Autodesk Inventor part; units mm, degrees
ref_plane "YZ Plane" through (0, 0, 0) normal (1, 0, 0) x (0, 1, 0)
ref_plane "XZ Plane" through (0, 0, 0) normal (0, 1, 0) x (-1, 0, 0)
ref_plane "XY Plane" through (0, 0, 0) normal (0, 0, 1) x (1, 0, 0)
sketch "Sketch4" plane through (0, 0, 0) normal (0, 0, 1) x (1, 0, 0)
  line L0 (1.3586, -0.1628) -> (1.3586, 19.8372)
  line L1 (1.3586, 19.8372) -> (26.3586, 19.8372)
  line L2 (26.3586, 19.8372) -> (36.8586, 14.8372)
  line L3 (36.8586, 14.8372) -> (173.3586, 14.8372)
  line L4 (173.3586, 14.8372) -> (173.3586, -50.1628)
  line L5 (173.3586, -50.1628) -> (153.3586, -50.1628)
  line L6 (153.3586, -50.1628) -> (153.3586, -5.1628)
  line L7 (153.3586, -5.1628) -> (36.8586, -5.1628)
  line L8 (36.8586, -5.1628) -> (26.3586, -0.1628)
  line L9 (26.3586, -0.1628) -> (1.3586, -0.1628)
  dimension "d55" = 20
  dimension "d56" = 25
  dimension "d57" = 5
  dimension "d58" = 20
  dimension "d59" = 45
  dimension "d60" = 152
  dimension "d61" = 10.5
extrude "Arm Base" add sketch "Sketch4" along normal blind 10
sketch "Sketch5" plane through (0, 0, 10) normal (0, 0, 1) x (1, 0, 0)
  line L0 (153.3586, -50.1628) -> (173.3586, -50.1628)
  line L1 (153.3586, -5.1628) -> (153.3586, -50.1628)
  point P0 (163.3586, -40.1628)
  dimension "d62" = 10
  dimension "d63" = 10
hole "Pivot Holes" at (163.3586, -40.1628, 10) direction (0, 0, -1) diameter 8 end through all
sketch "Sketch6" plane through (0, 0, 10) normal (0, 0, 1) x (1, 0, 0)
  line L0 (7.8586, 13.3372) -> (14.8586, 13.3372)
  line L1 (14.8586, 13.3372) -> (14.8586, 6.3372)
  line L2 (14.8586, 6.3372) -> (7.8586, 6.3372)
  line L3 (7.8586, 6.3372) -> (7.8586, 13.3372)
  line L4 (1.3586, 19.8372) -> (1.3586, -0.1628)
  point P0 (0, 0)
  point P1 (7.8586, 9.8372)
  point P2 (1.3586, 9.8372)
  dimension "d48" = 7
  dimension "d64" = 6.5
extrude "Extrusion5" cut sketch "Sketch6" against normal up to next
fillet "Fillet2" radius 10 5 edges at (1.3586, -0.1628, 5) (1.3586, 19.8372, 5) (173.3586, -50.1628, 5) (153.3586, -50.1628, 5) (173.3586, 14.8372, 5)
fillet "Fillet3" radius 2 26 edges at (170.4298, 11.9084, 10) (173.3586, -17.6628, 10) (170.4298, -47.234, 10) (153.3586, -22.6631, 10) (100.1089, 14.8372, 10) (95.1086, -5.1628, 10) (170.4298, -47.234, 0) (153.3586, -22.6631, 0) (170.4298, 11.9084, 0) (100.1089, 14.8372, 0) (173.3586, -17.6628, 0) (95.1086, -5.1628, 0) (18.8584, -0.1628, 0) (18.8584, 19.8372, 0) (4.2874, 2.766, 0) (18.8584, 19.8372, 10) (18.8584, -0.1628, 10) (4.2874, 2.766, 10) (31.6086, 17.3372, 10) (31.6086, -2.6628, 10) (31.6086, -2.6628, 0) (31.6086, 17.3372, 0) (26.3586, 19.8372, 5) (36.8586, 14.8372, 5) (26.3586, -0.1628, 5) (36.8586, -5.1628, 5)
fillet "Fillet4" radius 1 2 edges at (163.3586, -36.1628, 10) (163.3586, -36.1628, 0)
fillet "Fillet5" radius 1 8 edges at (7.8586, 9.8372, 10) (11.3586, 13.3372, 10) (14.8586, 9.8372, 10) (11.3586, 6.3372, 10) (7.8586, 9.8372, 0) (11.3586, 6.3372, 0) (14.8586, 9.8372, 0) (11.3586, 13.3372, 0)
properties part number "Lift Arm Lower"
The listing builds one solid part. Answer for the finished solid, in the listing's coordinates (mm). A direction names the side the tool comes from. Coordinates: 2 decimals unless noted, no trailing zeros. Write each loop counter-clockwise with the first axis right and the second up, starting at its lowest first coordinate (ties: lowest second). Pieces come first, ordered by that corner, then holes. Notation, with made-up numbers: (59, 74) - (79, 74) arc R17 ccw to (79, 78) - close; hole circle Ø8 at (-12.5, 44.5). An arc over 180 degrees is marked (long way). Return JSON: item names as keys, results as strings. Group by question number.
Q1. Find the intervals of material crossed by line 1 along X through (y, z) = (-40, 3.75); line 2 along X through (y, z) = (-6.5, 7.25); line 3 along X through (y, z) = (-36.5, 2.25), in increasing order. Write a range as [from, to].
Q2. Flat-ended cylindrical pins translate along their axes: pin 1 Ø5 at (x, z) = (92.5, 6) entering from -Y; pin 2 Ø1.8 at (y, z) = (-21, 6) entering from -X; pin 3 Ø3.5 at (x, z) = (13, 5.5) entering from -Y; pin 4 Ø5.5 at (y, z) = (9.5, 5) entering from -X. Find the tip coordinate at first contact, or state that the pin passes through.
Q3. The part is cut by section B-B on z = 5.5. State how many separate pieces and enclosed holes the cut face has, and give its area (3 significant figures).
Q4. Which of the six approach directions +Z, -Z, +X, -X, +Y, -Y give full straight-line access (tool end or side, diameter ignored) to faces 5 (the cylindrical face through (31.8, -2.09, 0.57)), 6 (the flat face through (153.359, -23, 5))?
Q5. The part is cut by section A-A on y = -16. Write down the section's boundary in (x, z).
Q6. For a pull along Y with two mould halves and no side action, classify faces 1 (the flat face through (31.676, -2.695, 4.958)), 2 (the cylindrical face through (167.263, -39.296, 4.944)), 3 (the cylindrical face through (31.43, 16.79, 9.4)), 4 (the flat face through (11, 6.337, 5)) as +Y half, -Y half, draft (parallel to the pull), parting line (faces both ways), or undercut.
Q7. The part is cut by section C-C on x = 18.5. Write down the section's boundary in (y, z), and give its area (3 significant figures).
Evaluation:
{
 "1": {"line 1": "x = [153.36, 159.36], [167.36, 173.36]", "line 2": "x = [153.36, 173.36]", "line 3": "x = [153.36, 161.75], [164.97, 173.36]"},
 "2": {"pin 1": "stops at y = -5.16", "pin 2": "stops at x = 153.36", "pin 3": "stops at y = -0.16", "pin 4": "stops at x = 1.36"},
 "3": {"separate pieces": "1", "enclosed holes": "2", "area": "4,130 mm2"},
 "4": {"face 5": "-Z, -X, -Y", "face 6": "+Z, -Z, -X, -Y"},
 "5": {"outline": "(153.36, 2) arc R2 ccw to (155.36, 0) - (171.36, 0) arc R2 ccw to (173.36, 2) - (173.36, 8) arc R2 ccw to (171.36, 10) - (155.36, 10) arc R2 ccw to (153.36, 8) - close"},
 "6": {"face 1": "-Y half", "face 2": "undercut", "face 3": "+Y half", "face 4": "undercut"},
 "7": {"outline": "(-0.16, 2) arc R2 ccw to (1.84, 0) - (17.84, 0) arc R2 ccw to (19.84, 2) - (19.84, 8) arc R2 ccw to (17.84, 10) - (1.84, 10) arc R2 ccw to (-0.16, 8) - close", "area": "197 mm2"}
}
